Autodesk Inventor part; units mm, degrees
ref_plane "YZ Plane" through (0, 0, 0) normal (1, 0, 0) x (0, 1, 0)
ref_plane "XZ Plane" through (0, 0, 0) normal (0, 1, 0) x (-1, 0, 0)
ref_plane "XY Plane" through (0, 0, 0) normal (0, 0, 1) x (1, 0, 0)
sketch "Sketch1" plane through (0, 0, 0) normal (0, 1, 0) x (-1, 0, 0)
  line L0 (-12.7, 69.85) -> (12.7, 69.85)
  line L1 (12.7, -69.85) -> (-12.7, -69.85)
  line L2 (-12.7, 69.85) -> (12.7, -69.85) construction
  line L3 (12.7, 69.85) -> (-12.7, -69.85) construction
  line L4 (30.48, 12.7) -> (30.48, -12.7)
  line L5 (-30.48, -12.7) -> (-30.48, 12.7)
  line L6 (-30.48, 12.7) -> (30.48, -12.7) construction
  line L7 (30.48, 12.7) -> (-30.48, -12.7) construction
  circle A0 centre (0, 0) radius 3.175
  line L8 (0, 64.77) -> (0, 9.525) construction
  line L9 (-2.413, 62.357) -> (-2.413, 11.938)
  line L10 (2.413, 11.938) -> (2.413, 62.357)
  arc A1 (2.413, 62.357) -> (-2.413, 62.357) centre (0, 62.357) ccw
  arc A2 (-2.413, 11.938) -> (2.413, 11.938) centre (0, 11.938) ccw
  line L11 (25.908, 0) -> (9.017, 0) construction
  line L12 (23.495, 2.413) -> (11.43, 2.413)
  line L13 (11.43, -2.413) -> (23.495, -2.413)
  arc A3 (23.495, -2.413) -> (23.495, 2.413) centre (23.495, 0) ccw
  arc A4 (11.43, 2.413) -> (11.43, -2.413) centre (11.43, 0) ccw
  line L14 (-2.413, -62.357) -> (-2.413, -11.938)
  line L15 (2.413, -11.938) -> (2.413, -62.357)
  arc A5 (-2.413, -62.357) -> (2.413, -62.357) centre (0, -62.357) ccw
  arc A6 (2.413, -11.938) -> (-2.413, -11.938) centre (0, -11.938) ccw
  line L16 (-23.495, 2.413) -> (-11.43, 2.413)
  line L17 (-11.43, -2.413) -> (-23.495, -2.413)
  arc A7 (-23.495, 2.413) -> (-23.495, -2.413) centre (-23.495, 0) ccw
  arc A8 (-11.43, -2.413) -> (-11.43, 2.413) centre (-11.43, 0) ccw
  line L18 (12.7, 12.7) -> (30.48, 12.7)
  line L19 (12.7, 69.85) -> (12.7, 12.7)
  line L20 (12.7, -12.7) -> (12.7, -69.85)
  line L21 (-12.7, -12.7) -> (-30.48, -12.7)
  line L22 (30.48, -12.7) -> (12.7, -12.7)
  line L23 (-30.48, 12.7) -> (-12.7, 12.7)
  line L24 (-12.7, 12.7) -> (-12.7, 69.85)
  line L25 (-12.7, -69.85) -> (-12.7, -12.7)
  point P0 (0, 37.1475)
  point P1 (17.4625, 0)
  dimension "d0" = 25.4
  dimension "d1" = 139.7
  dimension "d2" = 60.96
  dimension "d3" = 25.4
  dimension "d4" = 6.35
  dimension "d5" = 4.826
  dimension "d6" = 4.826
  dimension "d7" = 5.08
  dimension "d8" = 9.525
  dimension "d9" = 4.572
  dimension "d10" = 9.017
extrude "Extrusion1" add sketch "Sketch1" along normal blind 5.08
fillet "Fillet1" radius 3.175 12 edges at (12.7, 2.54, 69.85) (-12.7, 2.54, 69.85) (12.7, 2.54, 12.7) (30.48, 2.54, 12.7) (30.48, 2.54, -12.7) (12.7, 2.54, -12.7) (-12.7, 2.54, -12.7) (-12.7, 2.54, 12.7) (-30.48, 2.54, 12.7) (-30.48, 2.54, -12.7) (-12.7, 2.54, -69.85) (12.7, 2.54, -69.85)
properties part number "inertiabar"
The listing builds one solid part. Answer for the finished solid, in the listing's coordinates (mm). A direction names the side the tool comes from. Give positions to 0.01 mm unless a question says otherwise; leave off trailing zeros. Write each loop counter-clockwise with the first axis right and the second up, starting at its lowest first coordinate (ties: lowest second). Pieces come first, ordered by that corner, then holes. Notation, with made-up numbers: (-8.5, 2.25) -> (29.5, 2.25) arc R21 cw to (29.5, 41.25) -> close; hole circle Ø7 at (57.5, 84). An arc over 180 degrees is marked (long way). Use one line per item in the form item = value.
1) Section A-A on z = -18 is taken. Write down the section's boundary in (x, y), plus the area to 3 significant figures.
Result:
outline = (-12.7, 0) -> (-2.41, 0) -> (-2.41, 5.08) -> (-12.7, 5.08) -> close; (2.41, 0) -> (12.7, 0) -> (12.7, 5.08) -> (2.41, 5.08) -> close
area = 105 mm²
2) Section B-B on z = 0 is taken. Write down the section's boundary in (x, y) (3 decimals).
Result:
outline = (-30.48, 0) -> (-25.908, 0) -> (-25.908, 5.08) -> (-30.48, 5.08) -> close; (-9.017, 0) -> (-3.175, 0) -> (-3.175, 5.08) -> (-9.017, 5.08) -> close; (3.175, 0) -> (9.017, 0) -> (9.017, 5.08) -> (3.175, 5.08) -> close; (25.908, 0) -> (30.48, 0) -> (30.48, 5.08) -> (25.908, 5.08) -> close
3) Section C-C on y = 2.35 is taken. Count the separate pieces of the cut face and the enclosed holes in it, plus the area to 3 significant figures.
Result:
separate_pieces = 1
enclosed_holes = 5
area = 3,740 mm²
4) Each of these flat-tipped pins is pushed along its axis until it touches: P1, Ø2.5, axis at x = 14.5, y = 2, coming from the -Z side; P2, Ø1.5, axis at x = -15.5, y = 3, coming from the -Z side; P3, Ø2, axis at y = 3, z = 50.5, coming from the -X side; P4, Ø5.5, axis at x = 0, z = 0, coming from the -Y side. Where does it stop, or does it pass through?
Result:
P1 = -14.09
P2 = -12.91
P3 = -12.7
P4 = through
5) For a pull along X with two mould halves and no side action, classify faces 4 (the flat face through (-30.48, 3, 0)), 5 (the flat face through (2.413, 3, -38)), 6 (the cylindrical face through (13.61, 2.58, -13.65)) as +X half, -X half, draft (parallel to the pull), parting line (faces both ways), or undercut.
Result:
face_4 = -X half
face_5 = undercut
face_6 = +X half
6) Straight lines are drawn through the part: probe 1 along Z at (x, y) = (0, 1.1) (3 decimals); probe 2 along X at (y, z) = (3.2, -2); probe 3 along X at (y, z) = (4, -38.5). For each, find the intervals that lie inside material, in ascending order.
Result:
probe_1 = -69.85 to -64.77, -9.525 to -3.175, 3.175 to 9.525, 64.77 to 69.85
probe_2 = -30.48 to -24.85, -10.08 to -2.47, 2.47 to 10.08, 24.85 to 30.48
probe_3 = -12.7 to -2.41, 2.41 to 12.7
7) A tool of negligible diameter and unlimited length cuts with its end or side. For faces 1 (the flat face through (18, 3, 2.413)), 2 (the flat face through (22, 3, 12.7)), 3 (the flat face through (-22, 3, 12.7)), from which of +Z, -Z, +X, -X, +Y, -Y can it reach the whole face along a straight path? Write none if from no direction.
Result:
face_1 = +Y, -Y
face_2 = +Z, +X, +Y, -Y
face_3 = +Z, -X, +Y, -Y
